Could you check a few things on this drawing? It's one solid part, dimensions in mm from its lowest x, y, z. A direction names the side the tool comes from. Give positions to 0.01 mm unless a question says otherwise; leave off trailing zeros. Order: outer loops, then holes, each group sorted by start corner. A loop starts at its lowest first (then second) coordinate and runs counter-clockwise, first axis right, second up.
(1) Imagine slicing it at A-A, the plane x = 14.75. Write out the boundary of the cut face in (y, z), then the cut area to 3 significant figures.
(2) Imagine slicing it at C-C, the plane z = 16. Write out the boundary of the cut face in (x, y) (3 decimals).
(3) Imagine slicing it at D-D, the plane z = 29.5. Write out the boundary of the cut face in (x, y), then the cut area to 3 significant figures.
(4) On a 3-axis mill with a long thin cutter (end or side, diameter ignored), from which of +Z, -Z, +X, -X, +Y, -Y can I reach the whole of each face in a straight line? I mean the marked faces 1, 2 and 3. Say none if no direction works.
(5) If I drill on probe 1 along X at (y, z) = (15.5, 8); probe 2 along Y at (x, z) = (16.5, 8); probe 3 along Z at (x, y) = (11.5, 23), over which ranges is the centre line in solid material (lowest first)?
(6) Will these pins go through, and if not, where does the flat tip stop? pin 1 (8 mm diameter, centred on y = 26, z = 21.5, fed in from +X); pin 2 (2.5 mm diameter, centred on y = 15.5, z = 6, fed in from +X); pin 3 (4 mm diameter, centred on x = 13, z = 4.5, fed in from +Y).
(7) Imagine slicing it at B-B, the plane z = 3. Write out the boundary of the cut face in (x, y), then the cut area to 3 significant figures.
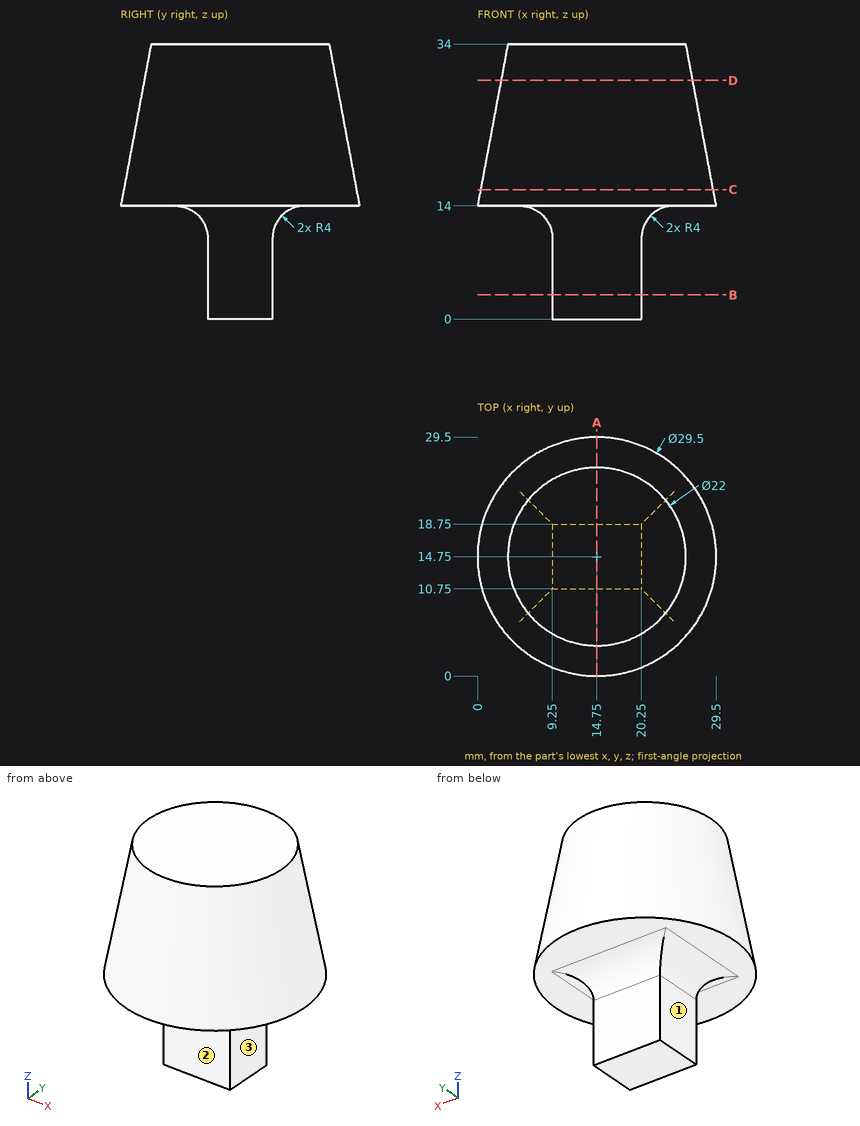
Answer block:
1. outline: (0, 14) - (6.75, 14) arc R4 cw to (10.75, 10) - (10.75, 0) - (18.75, 0) - (18.75, 10) arc R4 cw to (22.75, 14) - (29.5, 14) - (25.75, 34) - (3.75, 34) - close
1. area: 634 mm2
2. outline: circle Ø28.75 at (14.75, 14.75)
3. outline: circle Ø23.69 at (14.75, 14.75)
3. area: 441 mm2
4. face 1: -Z, -X, +Y, -Y
4. face 2: -Z, +X, -X, -Y
4. face 3: -Z, +X, +Y, -Y
5. probe 1: x = 9.25 to 20.25
5. probe 2: y = 10.75 to 18.75
5. probe 3: z = 14 to 34
6. pin 1: stops at x = 26.1
6. pin 2: stops at x = 20.25
6. pin 3: stops at y = 18.75
7. outline: (9.25, 10.75) - (20.25, 10.75) - (20.25, 18.75) - (9.25, 18.75) - close
7. area: 88.0 mm2
